The model under review builds one solid part; all positions refer to its coordinate system, in mm. A direction names the side the tool comes from. Coordinates: 2 decimals unless noted, no trailing zeros. Order: outer loops, then holes, each group sorted by start corner. A loop starts at its lowest first (then second) coordinate and runs counter-clockwise, first axis right, second up. Notation, with made-up numbers: M 52,84 L 86,84 A20 ccw 86,104 Z; hole C 33.5,65 d7. An arc over 180 degrees is marked long. Write each question's results on one line, items separated by ' | '.
from build123d import *

# Parameters (mm, degrees)
SKETCH_1_W          = 7.8
SKETCH_1_H          = 44
EXTRUDE_1_DEPTH     = 3
SKETCH_2_W          = 7.8
SKETCH_2_H          = 7
EXTRUDE_2_DEPTH     = 2
EXTRUDE_3_DEPTH     = 2
EXTRUDE_4_DEPTH     = 2
SKETCH_6_W          = 46.213242819
SKETCH_6_H          = 7
EXTRUDE_5_DEPTH     = 1
SKETCH_7_W          = 3
SKETCH_7_H          = 6
CUT_EXTRUDE_1_DEPTH = 3
SKETCH_8_W          = 6
SKETCH_8_H          = 3
CUT_EXTRUDE_2_DEPTH = 3


with BuildPart() as part:
    # 草图1 → 凸台-拉伸1 (new body)
    with BuildSketch(Plane(origin=(0, 0, 0), x_dir=(1, 0, 0), z_dir=(0, 1, 0))):
        with Locations((-7.618235554, 22)):
            Rectangle(SKETCH_1_W, SKETCH_1_H)
    extrude(amount=EXTRUDE_1_DEPTH)

    # 草图2 → 凸台-拉伸2 (add)
    with BuildSketch(Plane(origin=(0, 0, -44), x_dir=(-1, 0, 0), z_dir=(0, 0, -1))):
        with Locations((7.618235554, 3.5)):
            Rectangle(SKETCH_2_W, SKETCH_2_H)
    extrude(amount=EXTRUDE_2_DEPTH)

    # 草图4 → 凸台-拉伸3 (add)
    with BuildSketch(Plane(origin=(-3.718235554, 0, 0), x_dir=(0, 0, -1), z_dir=(1, 0, 0))):
        Polygon((46, 7), (44, 7), (40, 3), (40, 0), (46, 0), align=None)
    extrude(amount=EXTRUDE_3_DEPTH)

    # 草图5 → 凸台-拉伸4 (add)
    with BuildSketch(Plane(origin=(-3.718235554, 0, 0), x_dir=(0, 0, -1), z_dir=(1, 0, 0))):
        Polygon((0, 0), (0, 7), (4, 3), (4, 0), align=None)
    extrude(amount=EXTRUDE_4_DEPTH)

    # 草图6 → 凸台-拉伸5 (add)
    with BuildSketch(Plane.ZY.offset(11.518235554)):
        with Locations((-22.89337859, 3.5)):
            Rectangle(SKETCH_6_W, SKETCH_6_H)
    extrude(amount=EXTRUDE_5_DEPTH)

    # 草图7 → 切除-拉伸1 (cut)
    with BuildSketch(Plane.XZ):
        with Locations((-7.218235554, -23)):
            Rectangle(SKETCH_7_W, SKETCH_7_H)
    extrude(amount=-CUT_EXTRUDE_1_DEPTH, mode=Mode.SUBTRACT)

    # 草图8 → 切除-拉伸2 (cut)
    with BuildSketch(Plane.XZ):
        with Locations((-7.218235554, -23)):
            Rectangle(SKETCH_8_W, SKETCH_8_H)
    extrude(amount=-CUT_EXTRUDE_2_DEPTH, mode=Mode.SUBTRACT)


solid = part.part
1) The part is to be moulded in two halves that separate along X. For faces 1 (the flat face through (-12.518, 4, -23)), 2 (the flat face through (-12, 7, -30)), 3 (the flat face through (-5.718, 1, -21)), say which applies: pulls with the +X half, pulls with the -X half, needs draft (parallel to the pull), parting line crosses it, or undercut.
Solutions:
face 1: pulls with the -X half | face 2: needs draft | face 3: undercut
2) For pin 1 (3.5 mm diameter, centred on y = 2, z = -26.5, fed in from +X); pin 2 (1.5 mm diameter, centred on x = -9, z = -15.5, fed in from +Y); pin 3 (1.2 mm diameter, centred on x = -10, y = 2, fed in from +Z), all flat-tipped, find the tip position at first contact; note any pin that passes through.
Solutions:
pin 1: x = -3.72 | pin 2: y = 3 | pin 3: z = 0
3) Take a section at B-B on x = -7. State the section outline as (y, z) points, plus the area to 3 significant figures.
Solutions:
outline: M 0,-46 L 7,-46 L 7,-44 L 3,-44 L 3,-26 L 0,-26 Z; M 0,-20 L 3,-20 L 3,0 L 0,0 Z | area: 128 mm2
4) Take a section at C-C on z = -2.5. State the section outline as (x, y) points.
Solutions:
outline: M -12.52,0 L -1.72,0 L -1.72,4.5 L -3.72,4.5 L -3.72,3 L -11.52,3 L -11.52,7 L -12.52,7 Z
5) Take a section at A-A on y = 5.75. State the section outline as (x, z) points.
Solutions:
outline: M -12.52,-46 L -1.72,-46 L -1.72,-42.75 L -3.72,-42.75 L -3.72,-44 L -11.52,-44 L -11.52,0.21 L -12.52,0.21 Z; M -3.72,-1.25 L -1.72,-1.25 L -1.72,0 L -3.72,0 Z
6) To check wall thickness, follow line 1 along Z through (x, y) = (-3.5, 1); line 2 along X through (y, z) = (0.5, -23); line 3 along Z through (x, y) = (-5.75, 6.25). State the ranges of each line that lie inside material, in increasing order.
Solutions:
line 1: -46 to -40, -4 to 0 | line 2: -12.52 to -10.22, -4.22 to -3.72 | line 3: -46 to -44
7) For faces 4 (the flat face through (-3, 2, -40)), 5 (the flat face through (-11, 3, -22)), 6 (the flat face through (-3, 5, -2)), 7 (the flat face through (-7, 1, -20)), list the 3-axis set-ups (+Z, -Z, +X, -X, +Y, -Y) from which the entire face can be reached by the end or side of a thin tool; tool diameter is ignored.
Solutions:
face 4: +X, +Y, -Y | face 5: +Z, +Y | face 6: +X, +Y | face 7: +Y, -Y
8) Take a section at D-D on y = 2.5. State the section outline as (x, z) points.
Solutions:
outline: M -12.52,-46 L -1.72,-46 L -1.72,-40 L -3.72,-40 L -3.72,-4 L -1.72,-4 L -1.72,0 L -11.52,0 L -11.52,0.21 L -12.52,0.21 Z; hole M -10.22,-24.5 L -8.72,-24.5 L -8.72,-26 L -5.72,-26 L -5.72,-24.5 L -4.22,-24.5 L -4.22,-21.5 L -5.72,-21.5 L -5.72,-20 L -8.72,-20 L -8.72,-21.5 L -10.22,-21.5 Z
